The listing builds one solid part. Answer for the finished solid, in the listing's coordinates (mm). A direction names the side the tool comes from. Give positions to 0.01 mm unless a question says otherwise; leave off trailing zeros. Write each loop counter-clockwise with the first axis right and the second up, starting at its lowest first coordinate (ties: lowest second). Pieces come first, ordered by that corner, then holes. Notation, with made-up numbers: (37, -25) - (52, -25) arc R17 cw to (52, -9) - close; hole circle Ø11 at (-27, -23). An arc over 180 degrees is marked (long way). Write each question's results on one line, items separated by ' | '. Start each with the question number.
Q1. Section C-C (y = 17.5) is taken. Determine the outline of the cut face in (x, z).
Q2. For faces 5 (the face through (-143, 23.33, 12)), 6 (the face through (-130.88, 13, 23)), 7 (the face through (-9.5, 8, -66.3)), 8 (the face through (-130.88, 33, -39)), determine the directions among +Z, -Z, +X, -X, +Y, -Y from which every point of the face is accessible in a straight line to the end or side of a thin tool.
Q3. Section B-B (x = -84) is taken. Determine the outline of the cut face in (y, z), plus the area to 3 significant figures.
Q4. Flat-ended cylindrical pins translate along their axes: pin 1 Ø25 at (x, z) = (-151, -32.5) entering from +Y; pin 2 Ø1.8 at (x, z) = (-143, -87.5) entering from +Y; pin 3 Ø8 at (x, y) = (-14.5, 28) entering from +Z. Find the tip coordinate at first contact, or state that the pin passes through.
Q5. Find the intervals of material crossed by probe 1 along Z at (x, y) = (-11.18, 4); probe 2 along Z at (x, y) = (-100, 12); probe 3 along X at (y, z) = (24.2, -62.98) (3 decimals), in increasing order.
Q6. For a pull along Z with two mould halves and no side action, classify faces 1 (the face through (-105, 0, -37)), 2 (the face through (-6.879, 3.944, -6.104)), 3 (the face through (-57, 20, 10)), 4 (the face through (-57, 20, -85.69)) as pulls with the +Z half, pulls with the -Z half, needs draft (parallel to the pull), parting line crosses it, or undercut.
Q7. Section D-D (z = -78.5) is taken. Determine the outline of the cut face in (x, y).
Q8. Section A-A (z = -37.98) is taken. Determine the outline of the cut face in (x, y) (3 decimals), plus the area to 3 significant figures.
```python
from build123d import *

# Parameters (mm, degrees)
SKETCH8_W           = 131.76
SKETCH8_H           = 95.69
SKETCH8_R           = 3.43
SKETCH8_W_2         = 73.4
SKETCH8_H_2         = 33.99
BOSS_EXTRUDE4_DEPTH = 40
SKETCH9_R           = 8
CUT_EXTRUDE2_DEPTH  = 8
SKETCH12_W          = 9.12
SKETCH12_H          = 95.69
BOSS_EXTRUDE5_DEPTH = 40
BOSS_EXTRUDE6_DEPTH = 26.38
SKETCH15_R          = 3.05
CUT_EXTRUDE4_DEPTH  = 3.05
SKETCH14_R          = 3.05
CUT_EXTRUDE3_DEPTH  = 3.05


with BuildPart() as part:
    # Sketch8 → Boss-Extrude4 (new body)
    with BuildSketch(Plane(origin=(0, 0, 0), x_dir=(1, 0, 0), z_dir=(0, 1, 0))):
        with Locations((-55.88, 37.845)):
            Rectangle(SKETCH8_W, SKETCH8_H)
        with Locations((-100.58, 12.85)):
            Circle(SKETCH8_R, mode=Mode.SUBTRACT)
        with Locations((-100.58, 62.84)):
            Circle(SKETCH8_R, mode=Mode.SUBTRACT)
        with Locations((-11.18, 62.84)):
            Circle(SKETCH8_R, mode=Mode.SUBTRACT)
        with Locations((-11.18, 12.85)):
            Circle(SKETCH8_R, mode=Mode.SUBTRACT)
        with Locations((-55.88, 37.845)):
            Rectangle(SKETCH8_W_2, SKETCH8_H_2, mode=Mode.SUBTRACT)
    extrude(amount=BOSS_EXTRUDE4_DEPTH)

    # Sketch9 → Cut-Extrude2 (cut)
    with BuildSketch(Plane.XZ):
        with Locations((-100.58, -12.85)):
            Circle(SKETCH9_R)
        with Locations((-11.18, -12.85)):
            Circle(SKETCH9_R)
        with Locations((-11.18, -62.84)):
            Circle(SKETCH9_R)
        with Locations((-100.58, -62.84)):
            Circle(SKETCH9_R)
    extrude(amount=-CUT_EXTRUDE2_DEPTH, mode=Mode.SUBTRACT)

    # Sketch12 → Boss-Extrude5 (add)
    with BuildSketch(Plane.XZ):
        with Locations((-126.32, -37.845)):
            Rectangle(SKETCH12_W, SKETCH12_H)
        with Locations((14.56, -37.845)):
            Rectangle(SKETCH12_W, SKETCH12_H)
    extrude(amount=-BOSS_EXTRUDE5_DEPTH)

    # Sketch13 → Boss-Extrude6 (add)
    with BuildSketch(Plane.XZ):
        Polygon((-130.88, -85.69), (-130.88, 10), (-130.88, 37.02), (-180.93, 37.02), (-180.93, -112.98), (-130.88, -112.98), align=None)
    extrude(amount=-BOSS_EXTRUDE6_DEPTH)

    # Sketch15 → Cut-Extrude4 (cut)
    with BuildSketch(Plane(origin=(0, 26.38, 0), x_dir=(1, 0, 0), z_dir=(0, 1, 0))):
        with Locations((-168.4175, 87.98)):
            Circle(SKETCH15_R)
        with Locations((-143.3925, 87.98)):
            Circle(SKETCH15_R)
        with Locations((-155.905, 62.98)):
            Circle(SKETCH15_R)
        with Locations((-155.905, 37.98)):
            Circle(SKETCH15_R)
        with Locations((-155.905, 12.98)):
            Circle(SKETCH15_R)
        with Locations((-168.4175, -12.02)):
            Circle(SKETCH15_R)
        with Locations((-143.3925, -12.02)):
            Circle(SKETCH15_R)
    extrude(amount=-CUT_EXTRUDE4_DEPTH, mode=Mode.SUBTRACT)

    # Sketch14 → Cut-Extrude3 (cut)
    with BuildSketch(Plane(origin=(0, 26.38, 0), x_dir=(1, 0, 0), z_dir=(0, 1, 0))):
        with Locations((-105.88, -22.5125)):
            Circle(SKETCH14_R)
        with Locations((-105.88, -47.5375)):
            Circle(SKETCH14_R)
        with BuildLine():
            ThreePointArc((-77.83, -35.025), (-80.88, -31.975), (-83.93, -35.025))
            Line((-83.93, -35.025), (-77.83, -35.025))
        make_face()
        with BuildLine():
            Line((-77.83, -35.025), (-83.93, -35.025))
            ThreePointArc((-83.93, -35.025), (-80.88, -38.075), (-77.83, -35.025))
        make_face()
        with BuildLine():
            ThreePointArc((-52.83, -22.5125), (-53.723324317, -20.355824317), (-55.88, -19.4625))
            Line((-55.88, -19.4625), (-55.88, -25.5625))
            ThreePointArc((-55.88, -25.5625), (-53.723324317, -24.669175683), (-52.83, -22.5125))
        make_face()
        with BuildLine():
            Line((-55.88, -25.5625), (-55.88, -19.4625))
            ThreePointArc((-55.88, -19.4625), (-58.93, -22.5125), (-55.88, -25.5625))
        make_face()
        with BuildLine():
            ThreePointArc((-55.88, -44.4875), (-58.93, -47.5375), (-55.88, -50.5875))
            Line((-55.88, -50.5875), (-55.88, -44.4875))
        make_face()
        with BuildLine():
            Line((-55.88, -44.4875), (-55.88, -50.5875))
            ThreePointArc((-55.88, -50.5875), (-53.723324317, -49.694175683), (-52.83, -47.5375))
            ThreePointArc((-52.83, -47.5375), (-53.723324317, -45.380824317), (-55.88, -44.4875))
        make_face()
        with BuildLine():
            ThreePointArc((-33.93, -35.025), (-33.036675683, -37.181675683), (-30.88, -38.075))
            Line((-30.88, -38.075), (-30.88, -35.025))
            Line((-30.88, -35.025), (-33.93, -35.025))
        make_face()
        with BuildLine():
            Line((-30.88, -35.025), (-30.88, -38.075))
            ThreePointArc((-30.88, -38.075), (-28.723324317, -37.181675683), (-27.83, -35.025))
            Line((-27.83, -35.025), (-30.88, -35.025))
        make_face()
        with BuildLine():
            ThreePointArc((-27.83, -35.025), (-28.723324317, -32.868324317), (-30.88, -31.975))
            Line((-30.88, -31.975), (-30.88, -35.025))
            Line((-30.88, -35.025), (-27.83, -35.025))
        make_face()
        with BuildLine():
            Line((-30.88, -35.025), (-30.88, -31.975))
            ThreePointArc((-30.88, -31.975), (-33.036675683, -32.868324317), (-33.93, -35.025))
            Line((-33.93, -35.025), (-30.88, -35.025))
        make_face()
        with BuildLine():
            ThreePointArc((-2.83, -22.5125), (-3.723324317, -20.355824317), (-5.88, -19.4625))
            Line((-5.88, -19.4625), (-5.88, -25.5625))
            ThreePointArc((-5.88, -25.5625), (-3.723324317, -24.669175683), (-2.83, -22.5125))
        make_face()
        with BuildLine():
            Line((-5.88, -25.5625), (-5.88, -19.4625))
            ThreePointArc((-5.88, -19.4625), (-8.93, -22.5125), (-5.88, -25.5625))
        make_face()
        with BuildLine():
            ThreePointArc((-5.88, -44.4875), (-8.93, -47.5375), (-5.88, -50.5875))
            Line((-5.88, -50.5875), (-5.88, -44.4875))
        make_face()
        with BuildLine():
            Line((-5.88, -44.4875), (-5.88, -50.5875))
            ThreePointArc((-5.88, -50.5875), (-3.723324317, -49.694175683), (-2.83, -47.5375))
            ThreePointArc((-2.83, -47.5375), (-3.723324317, -45.380824317), (-5.88, -44.4875))
        make_face()
    extrude(amount=-CUT_EXTRUDE3_DEPTH, mode=Mode.SUBTRACT)


solid = part.part
```
Answers below:
1) outline: (-180.93, -112.98) - (-130.88, -112.98) - (-130.88, -85.69) - (19.12, -85.69) - (19.12, 10) - (-130.88, 10) - (-130.88, 37.02) - (-180.93, 37.02) - close; hole circle Ø6.86 at (-100.58, -62.84); hole circle Ø6.86 at (-100.58, -12.85); hole (-92.58, -54.84) - (-19.18, -54.84) - (-19.18, -20.85) - (-92.58, -20.85) - close; hole circle Ø6.86 at (-11.18, -62.84); hole circle Ø6.86 at (-11.18, -12.85)
2) face 5: +Y | face 6: +Z, +X, +Y, -Y | face 7: -Y | face 8: +Z, -Z, -X, +Y
3) outline: (0, -85.69) - (40, -85.69) - (40, -54.84) - (0, -54.84) - close; (0, -20.85) - (40, -20.85) - (40, 10) - (0, 10) - close | area: 2,470 mm2
4) pin 1: stops at y = 26.38 | pin 2: stops at y = 23.33 | pin 3: stops at z = 10
5) probe 1: z = -85.69 to -70.84, -54.84 to -20.85, -4.85 to 10 | probe 2: z = -85.69 to -66.22, -59.46 to -16.23, -9.47 to 10 | probe 3: x = -180.93 to -158.955, -152.855 to -104.007, -97.153 to -14.607, -7.753 to 19.12
6) face 1: needs draft | face 2: undercut | face 3: pulls with the +Z half | face 4: pulls with the -Z half
7) outline: (-180.93, 0) - (19.12, 0) - (19.12, 40) - (-130.88, 40) - (-130.88, 26.38) - (-180.93, 26.38) - close
8) outline: (-180.93, 0) - (-92.58, 0) - (-92.58, 40) - (-130.88, 40) - (-130.88, 26.38) - (-152.855, 26.38) - (-152.855, 23.33) - (-158.955, 23.33) - (-158.955, 26.38) - (-180.93, 26.38) - close; (-19.18, 0) - (19.12, 0) - (19.12, 40) - (-19.18, 40) - close | area: 4,370 mm2
